from build123d import *

# Parameters (mm, degrees)
ESQUISSE1_W        = 78
ESQUISSE1_H        = 62
BOSS_EXTRU_1_DEPTH = 9
CONG_1_R           = 17.5


with BuildPart() as part:
    # Esquisse1 → Boss.-Extru.1 (new body)
    with BuildSketch(Plane(origin=(0, 0, 0), x_dir=(1, 0, 0), z_dir=(0, 1, 0))):
        Rectangle(ESQUISSE1_W, ESQUISSE1_H)
    extrude(amount=BOSS_EXTRU_1_DEPTH)

    # Congé1
    cong_1_edges = [part.edges().sort_by_distance(p)[0] for p in [
        (-39, 4.5, -31),
        (39, 4.5, -31),
        (39, 4.5, 31),
        (-39, 4.5, 31),
    ]]
    fillet(cong_1_edges, radius=CONG_1_R)


solid = part.part
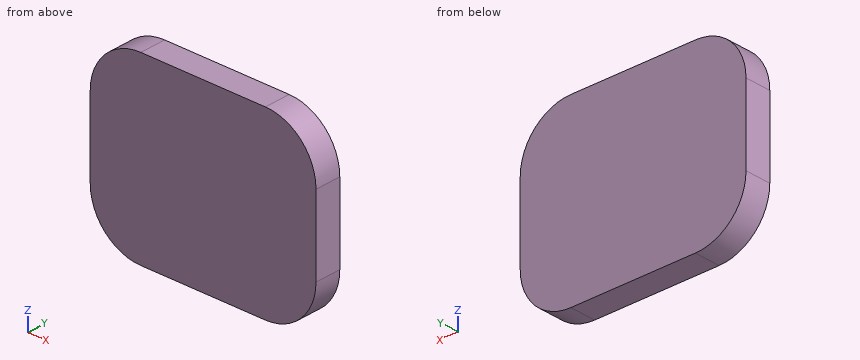
Could you check a few things on this model? Use its own coordinates, in mm. Give positions to 0.01 mm unless a question says otherwise; leave off trailing zeros. Order: outer loops, then holes, each group sorted by start corner. A loop starts at its lowest first (then second) coordinate and runs counter-clockwise, first axis right, second up.
1. Suppose I cut it at A-A (y = 6.5). Write out the boundary of the cut face in (x, z).
Answers below:
outline: (-39, -13.5) arc R17.5 ccw to (-21.5, -31) - (21.5, -31) arc R17.5 ccw to (39, -13.5) - (39, 13.5) arc R17.5 ccw to (21.5, 31) - (-21.5, 31) arc R17.5 ccw to (-39, 13.5) - close
2. Suppose I cut it at B-B (z = 24). Write out the boundary of the cut face in (x, y), plus the area to 3 significant figures.
Answers below:
outline: (-35.5, 0) - (35.5, 0) - (35.5, 9) - (-35.5, 9) - close
area: 639 mm2
3. For pin 1 (2 mm diameter, centred on y = 1, z = -20, fed in from -X); pin 2 (4 mm diameter, centred on x = 26, y = 2.5, fed in from -Z); pin 3 (3 mm diameter, centred on y = 1.5, z = 24.5, fed in from +X), each with a flat end and sliding along its axis, tell me the tip position at first contact or that it passes through.
Answers below:
pin 1: stops at x = -38.11
pin 2: stops at z = -30.82
pin 3: stops at x = 36.2
4. Suppose I cut it at C-C (x = 33). Write out the boundary of the cut face in (y, z), plus the area to 3 significant figures.
Answers below:
outline: (0, -26.69) - (9, -26.69) - (9, 26.69) - (0, 26.69) - close
area: 480 mm2
5. I need wall thicknesses on L1, parallel to Z at x = -30, y = 7.5; L2, parallel to X at y = 3.5, z = 28.5; L3, parallel to X at y = 7.75, z = 23. Which ranges of each line are inside material? Lowest first, please.
Answers below:
L1: z = -28.8 to 28.8
L2: x = -30.51 to 30.51
L3: x = -36.2 to 36.2
